CAD build for the part. Positions are in the model's coordinates, mm. A direction names the side the tool comes from. Give positions to 0.01 mm unless a question says otherwise; leave off trailing zeros. Write each loop counter-clockwise with the first axis right and the second up, starting at its lowest first coordinate (ties: lowest second). Pieces come first, ordered by that corner, then holes. Notation, with made-up numbers: (-7.5, 11.25) - (6.5, 11.25) arc R30 ccw to (6.5, 42.25) - close; hole circle Ø10 at (62.5, 72). An arc over 180 degrees is marked (long way). Answer as a JSON object with one key per item and string values.
from build123d import *

# Parameters (mm, degrees)
SKETCH035_W             = 115
SKETCH035_H             = 110
PAD002_DEPTH            = 25
SKETCH036_W             = 115
SKETCH036_H             = 20
PAD003_DEPTH            = 68
SKETCH037_R             = 2.75
HOLE001_DEPTH           = 68.001
HOLE004_D               = 5.5
HOLE004_CBORE_D         = 13
HOLE004_CBORE_DEPTH     = 6.4
BODY008_PLACEMENT_ANGLE = 45


with BuildPart() as part:
    # Sketch035 → Pad002 (new body)
    with BuildSketch(Plane.XY.offset(-39)):
        with Locations((217.5, 35)):
            Rectangle(SKETCH035_W, SKETCH035_H)
    extrude(amount=-PAD002_DEPTH)

    # Sketch036 → Pad003 (join)
    with BuildSketch(Plane.XY.offset(4)):
        with Locations((217.5, -15)):
            Rectangle(SKETCH036_W, SKETCH036_H)
    extrude(amount=-PAD003_DEPTH)

    # Sketch037 → Hole001 (cut, through all)
    with BuildSketch(Plane.XY.offset(4)):
        with Locations((175, -15)):
            Circle(SKETCH037_R)
        with Locations((265, -15)):
            Circle(SKETCH037_R)
        with Locations((220, -15)):
            Circle(SKETCH037_R)
    extrude(amount=-HOLE001_DEPTH, mode=Mode.SUBTRACT)

    # Hole004 (through all)
    with Locations(Plane(origin=(0, 0, -64), x_dir=(1, 0, 0), z_dir=(0, 0, -1))):
        with Locations((167.5, -77.5), (267.5, -77.5)):
            CounterBoreHole(HOLE004_D / 2, HOLE004_CBORE_D / 2, HOLE004_CBORE_DEPTH)


with BuildPart() as part_1:
    # Body008 placement: moved
    add(part.part.moved(Location((182.5, 417.426407, 42.426407))).rotate(Axis((182.5, 417.426407, 42.426407), (1, 0, 0)), BODY008_PLACEMENT_ANGLE))


solid = part_1.part
(1) Saw through at B-B, the plane x = 373. Give the cut face in (y, z), and give its area (4 significant figures).
Answer key:
{"outline": "(396.92, 27.58) - (445, -20.51) - (526.32, 60.81) - (508.64, 78.49) - (441.47, 11.31) - (411.06, 41.72) - close", "area": "3,735 mm²"}
(2) 3-axis set-ups, long thin cutter, end or side, ignore diameter. For faces 4 (the face through (451.353, 514.935, 58.476)), 5 (the face through (399.195, 475.526, 45.372)), 6 (the face through (457.5, 462, 24)): which of +Z, -Z, +X, -X, +Y, -Y reach the whole face in a straight line?
Answer key:
{"face 4": "none", "face 5": "+Z, +X, -X", "face 6": "+Z, -Z, +X, +Y, -Y"}
(3) Flat gauge pins, fed straight in: P1, Ø1.5, axis at x = 355.5, z = 61.5, coming from the -Y side; P2, Ø12, axis at x = 366.5, y = 481, coming from the -Z side; P3, Ø3, axis at x = 369, y = 496, coming from the -Z side. Where does each tip first touch, or does it go through?
Answer key:
{"P1": "stops at y = 490.9", "P2": "stops at z = 9.49", "P3": "stops at z = 28.99"}
(4) Saw through at A-A, the plane z = 30. State how many separate pieces and enclosed holes the cut face has, and give its area (3 significant figures).
Answer key:
{"separate pieces": "2", "enclosed holes": "3", "area": "6,660 mm²"}
(5) Probe L1, parallel to X at y = 431, z = 6; L2, parallel to Y at x = 363, z = 27; L3, parallel to Y at x = 388.5, z = 40. List the from-to ranges inside material, lowest first. Write a range as [from, to].
Answer key:
{"L1": "x = [342.5, 355.01], [359.99, 400.01], [404.99, 445.01], [449.99, 457.5]", "L2": "y = [397.5, 425.78], [457.15, 492.51]", "L3": "y = [409.34, 412.78], [470.15, 505.51]"}
(6) Pull direction Y, two halves, no side cores. Call faces 1 (the face through (447.38, 505.7, 62.58)), 2 (the face through (399.195, 404.09, 34.747)), 3 (the face through (399.2, 517.36, 69.77)): pulls with the +Y half, pulls with the -Y half, needs draft (parallel to the pull), parting line crosses it, or undercut.
Answer key:
{"face 1": "undercut", "face 2": "pulls with the -Y half", "face 3": "pulls with the +Y half"}
